Geometry: final body of the model. Coordinates: model frame, mm. Give positions to 0.01 mm unless a question says otherwise; leave off trailing zeros. Order: outer loops, then holes, each group sorted by start corner. A loop starts at its lowest first (then second) coordinate and runs counter-clockwise, first axis right, second up. Notation, with made-up numbers: (6, 33) - (32, 33) arc R16 ccw to (32, 52) - close; hole circle Ø8 at (60.25, 47.25). An arc over 180 degrees is marked (long way). Use one line per item in the form item = value.
from build123d import *

# Parameters (mm, degrees)
BOSS_EXTRUDE1_DEPTH = 3
SKETCH2_W           = 3
SKETCH2_H           = 10
CUT_EXTRUDE1_DEPTH  = 82.449370777


with BuildPart() as part:
    # Sketch1 → Boss-Extrude1 (new body)
    with BuildSketch(Plane.XY):
        with BuildLine():
            Line((0, 0), (60, 0))
            Line((60, 0), (60, 25))
            ThreePointArc((60, 25), (30, 55), (0, 25))
            Line((0, 25), (0, 0))
        make_face()
        with BuildLine():
            Line((37.5, 20), (39, 20))
            Line((39, 20), (48.179870439, 22.594220254))
            ThreePointArc((48.179870439, 22.594220254), (50, 25), (48.179870439, 27.405779746))
            Line((48.179870439, 27.405779746), (39, 30))
            Line((39, 30), (37.5, 30))
            ThreePointArc((37.5, 30), (35.732233047, 30.732233047), (35, 32.5))
            Line((35, 32.5), (35, 34))
            Line((35, 34), (32.405779746, 43.179870439))
            ThreePointArc((32.405779746, 43.179870439), (30, 45), (27.594220254, 43.179870439))
            Line((27.594220254, 43.179870439), (25, 34))
            Line((25, 34), (25, 32.5))
            ThreePointArc((25, 32.5), (24.267766953, 30.732233047), (22.5, 30))
            Line((22.5, 30), (21, 30))
            Line((21, 30), (11.820129561, 27.405779746))
            ThreePointArc((11.820129561, 27.405779746), (10, 25), (11.820129561, 22.594220254))
            Line((11.820129561, 22.594220254), (21, 20))
            Line((21, 20), (22.5, 20))
            ThreePointArc((22.5, 20), (24.267766953, 19.267766953), (25, 17.5))
            Line((25, 17.5), (25, 16))
            Line((25, 16), (27.594220254, 6.820129561))
            ThreePointArc((27.594220254, 6.820129561), (30, 5), (32.405779746, 6.820129561))
            Line((32.405779746, 6.820129561), (35, 16))
            Line((35, 16), (35, 17.5))
            ThreePointArc((35, 17.5), (35.732233047, 19.267766953), (37.5, 20))
        make_face(mode=Mode.SUBTRACT)
    extrude(amount=BOSS_EXTRUDE1_DEPTH)

    # Sketch2 → Cut-Extrude1 (cut, through all)
    with BuildSketch(Plane(origin=(0, 0, 0), x_dir=(-1, 0, 0), z_dir=(0, 0, -1))):
        with Locations((-58.5, 12.5)):
            Rectangle(SKETCH2_W, SKETCH2_H)
        with Locations((-1.5, 12.5)):
            Rectangle(SKETCH2_W, SKETCH2_H)
    extrude(amount=-CUT_EXTRUDE1_DEPTH, mode=Mode.SUBTRACT)


solid = part.part
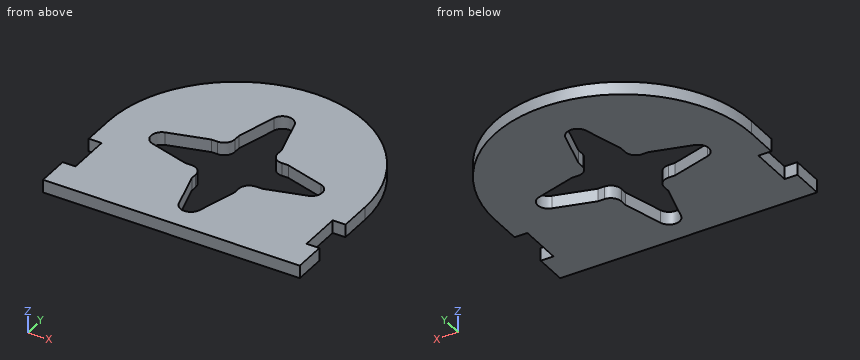
(1) Cut plane D-D on x = 5.5. Output: boundary loops of the cut face in (y, z), plus the area to 3 significant figures.
Computed values:
outline = (0, 0) - (42.31, 0) - (42.31, 3) - (0, 3) - close
area = 127 mm²
(2) Cut plane A-A on x = 30. Output: boundary loops of the cut face in (y, z).
Computed values:
outline = (0, 0) - (5, 0) - (5, 3) - (0, 3) - close; (45, 0) - (55, 0) - (55, 3) - (45, 3) - close
(3) Cut plane C-C on x = 53. Output: boundary loops of the cut face in (y, z), plus the area to 3 significant figures.
Computed values:
outline = (0, 0) - (44.26, 0) - (44.26, 3) - (0, 3) - close
area = 133 mm²
(4) Cut plane B-B on y = 37. Output: boundary loops of the cut face in (x, z).
Computed values:
outline = (2.5, 0) - (25.85, 0) - (25.85, 3) - (2.5, 3) - close; (34.15, 0) - (57.5, 0) - (57.5, 3) - (34.15, 3) - close
(5) Contact query for flat-ended pins moving along their axis: pin 1 Ø0.8 at (y, z) = (33.5, 1) entering from +X; pin 2 Ø0.8 at (y, z) = (17, 1.5) entering from +X; pin 3 Ø0.8 at (x, z) = (21.5, 2) entering from +Y. Output: stop coordinate, or through.
Computed values:
pin_1 = 58.89
pin_2 = 57
pin_3 = 53.89
(6) Ray query, line 1 along X through (y, z) = (16.5, 2.2); line 2 along Y through (x, z) = (41.5, 0.6); line 3 along X through (y, z) = (37.5, 1.4). Return the intervals inside material, ascending.
Computed values:
line_1 = 3 to 25, 35 to 57
line_2 = 0 to 20.71, 29.29 to 52.71
line_3 = 2.73 to 25.99, 34.01 to 57.27
